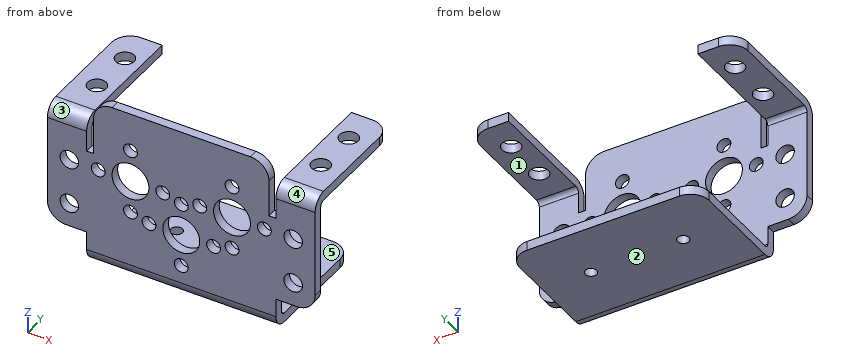
from build123d import *

# Parameters (mm, degrees)
T_LE_DE_BASE_PLI_E1_DEPTH             = 20.5
ESQUISSE8_W                           = 24
ESQUISSE8_H                           = 2
BOSS_EXTRU_1_DEPTH                    = 8.5
T_LE_PLI_E_SUR_AR_TE1_STRIP_W         = 10
T_LE_PLI_E_SUR_AR_TE1_STRIP_H         = 2
T_LE_PLI_E_SUR_AR_TE1_STRIP_CUT_DEPTH = 8.5
T_LE_PLI_E_SUR_AR_TE1_DEPTH           = 8.5
ESQUISSE12_W                          = 1.5
ESQUISSE12_H                          = 12
ENL_V_MAT_EXTRU_1_DEPTH               = 8.5
DIAM_TRE_DU_PER_AGE_4_0_4_1_D         = 4
DIAM_TRE_DU_PER_AGE_4_0_4_2_D         = 4
DIAM_TRE_DU_PER_AGE_2_5_2_5_2_D       = 2.5
CONG_1_R                              = 4
SKETCH1_R                             = 4
SKETCH1_R_2                           = 1.5
CUT_EXTRUDE1_DEPTH                    = 10


# Sheet-metal steps are written as plain solids
with BuildPart() as part:
    # Esquisse1 → Tôle de base pliée1 (new body)
    with BuildSketch(Plane(origin=(0, 0, 0), x_dir=(0, 0, -1), z_dir=(1, 0, 0))):
        with BuildLine():
            Line((0, 27), (0, 3))
            ThreePointArc((0, 3), (-0.878679656, 0.878679656), (-3, 0))
            Line((-3, 0), (-37.5, 0))
            Line((-37.5, 0), (-37.5, 2))
            Line((-37.5, 2), (-3, 2))
            ThreePointArc((-3, 2), (-2.292893219, 2.292893219), (-2, 3))
            Line((-2, 3), (-2, 27))
            Line((-2, 27), (0, 27))
        make_face()
    extrude(amount=T_LE_DE_BASE_PLI_E1_DEPTH)

    # Esquisse8 → Boss.-Extru.1 (add)
    with BuildSketch(Plane(origin=(20.5, 0, 0), x_dir=(0, 0, -1), z_dir=(1, 0, 0))):
        with Locations((-19, 1)):
            Rectangle(ESQUISSE8_W, ESQUISSE8_H)
    extrude(amount=BOSS_EXTRU_1_DEPTH)

    # Tôle pliée sur arête1 strip (across the edge) → Tôle pliée sur arête1 strip cut (cut)
    with BuildSketch(Plane(origin=(20.5, 2, 31), x_dir=(0, 0, -1), z_dir=(1, 0, 0))):
        with Locations((-4, -1)):
            Rectangle(T_LE_PLI_E_SUR_AR_TE1_STRIP_W, T_LE_PLI_E_SUR_AR_TE1_STRIP_H)
    extrude(amount=T_LE_PLI_E_SUR_AR_TE1_STRIP_CUT_DEPTH, mode=Mode.SUBTRACT)

    # Tôle pliée sur arête1 section (across the edge) → Tôle pliée sur arête1 (add)
    with BuildSketch(Plane(origin=(20.5, 2, 31), x_dir=(0, 0, -1), z_dir=(1, 0, 0))):
        with BuildLine():
            Line((-2, 1), (-2, 25))
            Line((-2, 25), (0, 25))
            Line((0, 25), (0, 1))
            ThreePointArc((0, 1), (0.292893219, 0.292893219), (1, 0))
            Line((1, 0), (1, -2))
            ThreePointArc((1, -2), (-1.121320344, -1.121320344), (-2, 1))
        make_face()
    extrude(amount=T_LE_PLI_E_SUR_AR_TE1_DEPTH)

    # Esquisse12 → Enlèv. mat.-Extru.1 (cut)
    with BuildSketch(Plane(origin=(0, 2, 0), x_dir=(1, 0, 0), z_dir=(0, 1, 0))):
        with Locations((19.75, -31.5)):
            Rectangle(ESQUISSE12_W, ESQUISSE12_H)
    extrude(amount=-ENL_V_MAT_EXTRU_1_DEPTH, mode=Mode.SUBTRACT)

    # Diamètre du perçage Ø4.0 (4)1 (through all)
    with Locations(Plane(origin=(0, 2, 0), x_dir=(1, 0, 0), z_dir=(0, 1, 0))):
        with Locations((24.25, -12.13), (24.25, -22.13)):
            Hole(DIAM_TRE_DU_PER_AGE_4_0_4_1_D / 2)

    # Diamètre du perçage Ø4.0 (4)2 (through all)
    with Locations(Plane.XY.offset(33)):
        with Locations((24.25, 19.87), (24.25, 9.87)):
            Hole(DIAM_TRE_DU_PER_AGE_4_0_4_2_D / 2)

    # Diamètre du perçage Ø2.5 (2.5)2 (through all)
    with Locations(Plane.XY.offset(2)):
        with Locations((10, 14.87)):
            Hole(DIAM_TRE_DU_PER_AGE_2_5_2_5_2_D / 2)

    # Congé1
    cong_1_edges = [part.edges().sort_by_distance(p)[0] for p in [
        (20.5, 27, 1),
        (29, 1, 7),
        (29, 27, 32),
        (19, 1, 37.5),
    ]]
    fillet(cong_1_edges, radius=CONG_1_R)

    # Symétrie1: part across plane


with BuildPart() as part_1:
    add(part.part)
    add(part.part.mirror(Plane(origin=(0, 3, 3), x_dir=(0, 0, 1), z_dir=(1, 0, 0))))

    # Sketch1 → Cut-Extrude1 (cut)
    with BuildSketch(Plane.XZ):
        with Locations(Location((0, 14, 0), (0, 0, 270))):
            Circle(SKETCH1_R)
        with Locations(Location((11, 22.13, 0), (0, 0, 270))):
            Circle(SKETCH1_R)
        with Locations(Location((-11, 22.13, 0), (0, 0, 270))):
            Circle(SKETCH1_R)
        with Locations(Location((4, 22.13, 0), (0, 0, 270))):
            Circle(SKETCH1_R_2)
        with Locations(Location((11, 29.13, 0), (0, 0, 270))):
            Circle(SKETCH1_R_2)
        with Locations(Location((18, 22.13, 0), (0, 0, 270))):
            Circle(SKETCH1_R_2)
        with Locations(Location((11, 15.13, 0), (0, 0, 270))):
            Circle(SKETCH1_R_2)
        with Locations(Location((-18, 22.13, 0), (0, 0, 270))):
            Circle(SKETCH1_R_2)
        with Locations(Location((0, 7, 0), (0, 0, 270))):
            Circle(SKETCH1_R_2)
        with Locations(Location((-11, 29.13, 0), (0, 0, 270))):
            Circle(SKETCH1_R_2)
        with Locations(Location((-4, 22.13, 0), (0, 0, 270))):
            Circle(SKETCH1_R_2)
        with Locations(Location((-11, 15.13, 0), (0, 0, 270))):
            Circle(SKETCH1_R_2)
        with Locations(Location((-7, 14, 0), (0, 0, 270))):
            Circle(SKETCH1_R_2)
        with Locations(Location((0, 21, 0), (0, 0, 270))):
            Circle(SKETCH1_R_2)
        with Locations(Location((7, 14, 0), (0, 0, 270))):
            Circle(SKETCH1_R_2)
    extrude(amount=-CUT_EXTRUDE1_DEPTH, mode=Mode.SUBTRACT)


solid = part_1.part
Design review of the part built by this model. Coordinates are the model's own, in mm. Face numbers are marked on the shaded views. A direction names the side the tool comes from. Coordinates: 2 decimals unless noted, no trailing zeros. Loops run counter-clockwise (first coordinate to the right, second up) from the corner with the lowest first, then second, coordinate; pieces in that order, holes last. Notation, with made-up numbers: (88.25, 23) - (112.25, 23) arc R20 cw to (112.25, 27) - close; hole circle Ø11 at (2.5, -0.5). An arc over 180 degrees is marked (long way). Use CSV: the item, a comma, the result in double quotes. Start each with the question number.
1. Add section B-B on z = 29.13. Give the boundary of the cut face in (x, y), plus the area to 3 significant figures.
2. Add section C-C on y = 9.87. Give the boundary of the cut face in (x, z), plus the area to 3 significant figures.
3. Add section A-A on y = 3.75. Give the boundary of the cut face in (x, z), plus the area to 3 significant figures.
4. For the marked faces 1, 2, 3, 4 and 5, list the 3-axis set-ups (+Z, -Z, +X, -X, +Y, -Y) from which the entire face can be reached by the end or side of a thin tool; tool diameter is ignored.
5. To check wall thickness, follow probe 1 along X at (y, z) = (1.3, 29.13); probe 2 along Y at (x, z) = (-21, 11.5). State the ranges of each line that lie inside material, in increasing order.
6. Clearance check with flat-ended pins moving along their axes: pin 1 (12 mm diameter, centred on x = -0.5, z = 28, fed in from -Y); pin 2 (8 mm diameter, centred on x = 6.5, z = 8, fed in from +Y); pin 3 (1.6 mm diameter, centred on x = -19.5, y = 1.5, fed in from +Z); pin 4 (4 mm diameter, centred on x = -25.5, y = 18, fed in from -Z). State where each tip first meets the part, or that it passes through.
7. Add section D-D on x = 18. Give the boundary of the cut face in (y, z), plus the area to 3 significant figures.
Resolved:
1,outline,"(-29, 0) - (-20.5, 0) - (-20.5, 2) - (-29, 2) - close; (-19, 0) - (-12.5, 0) - (-12.5, 2) - (-19, 2) - close; (-9.5, 0) - (9.5, 0) - (9.5, 2) - (-9.5, 2) - close; (12.5, 0) - (19, 0) - (19, 2) - (12.5, 2) - close; (20.5, 0) - (29, 0) - (29, 2) - (20.5, 2) - close"
1,area,"98.0 mm2"
2,outline,"(-29, 31) - (-26.25, 31) - (-26.25, 33) - (-29, 33) - close; (-22.25, 31) - (-20.5, 31) - (-20.5, 33) - (-22.25, 33) - close; (-20.5, 0) - (20.5, 0) - (20.5, 2) - (-20.5, 2) - close; (20.5, 31) - (22.25, 31) - (22.25, 33) - (20.5, 33) - close; (26.25, 31) - (29, 31) - (29, 33) - (26.25, 33) - close"
2,area,"100 mm2"
3,outline,"(-29, 31) - (-20.5, 31) - (-20.5, 33) - (-29, 33) - close; (-20.5, 0) - (20.5, 0) - (20.5, 2) - (-20.5, 2) - close; (20.5, 31) - (29, 31) - (29, 33) - (20.5, 33) - close"
3,area,"116 mm2"
4,face 1,"-Z, +X, -X, +Y"
4,face 2,"-Z, +X, -X, +Y, -Y"
4,face 3,"+Z, -X, -Y"
4,face 4,"+Z, +X, -Y"
4,face 5,"+Z, +X, -X, +Y"
5,probe 1,"-29 to -20.5, -19 to -12.5, -9.5 to 9.5, 12.5 to 19, 20.5 to 29"
5,probe 2,"0 to 2"
6,pin 1,"y = 0"
6,pin 2,"y = 2"
6,pin 3,"z = 35.02"
6,pin 4,"z = 31"
7,outline,"(0, 3) arc R3 ccw to (3, 0) - (26.71, 0) - (26.71, 2) - (3, 2) arc R1 cw to (2, 3) - (2, 20.63) - (0, 20.63) - close; (0, 23.63) - (2, 23.63) - (2, 36.15) - (0, 36.15) - close"
7,area,"114 mm2"
